Design review of the part built by this model. Coordinates are the model's own, in mm. Coordinates: 2 decimals unless noted, no trailing zeros. Order: outer loops, then holes, each group sorted by start corner. A loop starts at its lowest first (then second) coordinate and runs counter-clockwise, first axis right, second up.
from build123d import *

# Parameters (mm, degrees)
SKETCH_1_W          = 6.5
SKETCH_1_H          = 2
CUT_EXTRUDE_1_DEPTH = 1.5
CHAMFER_1_SIZE      = 0.75
CHAMFER_2_SIZE      = 0.6
CHAMFER_2_SIZE2     = 0.346410161
FILLET_1_R          = 0.1


with BuildPart() as part:
    # Эскиз1 → Повернуть1 (revolve)
    with BuildSketch(Plane(origin=(0, 0, 0), x_dir=(-1, 0, 0), z_dir=(0, 0, -1))):
        with Locations((-3.25, 1)):
            Rectangle(SKETCH_1_W, SKETCH_1_H)
    revolve(axis=Axis((6.5, 0, 0), (-1, 0, 0)))

    # Эскиз2 → Вырез-Вытянуть1 (cut)
    with BuildSketch(Plane.ZY):
        Polygon((1.154700538, 0), (0.577350269, 1), (-0.577350269, 1), (-1.154700538, 0), (-0.577350269, -1), (0.577350269, -1), align=None)
    extrude(amount=-CUT_EXTRUDE_1_DEPTH, mode=Mode.SUBTRACT)

    # Фаска1
    chamfer_1_edges = [part.edges().sort_by_distance(p)[0] for p in [
        (6.5, -2, 0),
    ]]
    chamfer(chamfer_1_edges, length=CHAMFER_1_SIZE)

    # Фаска2
    chamfer_2_edges = [part.edges().sort_by_distance(p)[0] for p in [
        (0, -2, 0),
    ]]
    chamfer_2_side = [part.faces().sort_by_distance(p)[0] for p in [
        (0, -1.943431458, 0),
    ]]
    chamfer(chamfer_2_edges, length=CHAMFER_2_SIZE, length2=CHAMFER_2_SIZE2, reference=chamfer_2_side[0])

    # Скругление1
    fillet_1_edges = [part.edges().sort_by_distance(p)[0] for p in [
        (1.5, -0.5, 0.866025404),
        (1.5, -1, 0),
        (1.5, -0.5, -0.866025404),
        (1.5, 0.5, -0.866025404),
        (1.5, 1, 0),
        (1.5, 0.5, 0.866025404),
        (0, -0.5, 0.866025404),
        (0, 0.5, 0.866025404),
        (0, 1, 0),
        (0, 0.5, -0.866025404),
        (0, -0.5, -0.866025404),
        (0, -1, 0),
        (0, -1.4, 0),
    ]]
    fillet(fillet_1_edges, radius=FILLET_1_R)


solid = part.part
1. Mouldability with a two-part tool opening along Y and no side actions: class faces 1 (the cylindrical face through (3, 0, 2)), 2 (the flat face through (0.74, -0.49, -0.87)), 3 (the flat face through (6.5, 0, 0)), 4 (the flat face through (0.74, 0.51, -0.86)) as pulls with the +Y half, pulls with the -Y half, needs draft (parallel to the pull), parting line crosses it, or undercut.
2. Add section C-C (x = 3). Give the boundary of the cut face in (y, z).
3. To check wall thickness, follow line 1 (Y direction, x = 1.25, z = -0.1); line 2 (Z direction, x = 0.5, y = -0.6); line 3 (X direction, y = 0.7, z = -0.65). State the ranges of each line that lie inside material, in increasing order.
4. Add section A-A (x = 0.75). Give the boundary of the cut face in (y, z).
5. Add section B-B (z = 0). Give the boundary of the cut face in (x, y), and give its area (3 significant figures).
6. Insertion check: pin 1 (1.5 mm diameter, centred on x = 5.5, y = 1, fed in from -Z); pin 2 (2 mm diameter, centred on x = 5, y = -1.5, fed in from +Z). Each pin has a flat end and moves straight along its axis. Give the tip position at first contact, or say it passes through.
Solution:
1. face 1: parting line crosses it
1. face 2: undercut
1. face 3: needs draft
1. face 4: undercut
2. outline: circle Ø4 at (0, 0)
3. line 1: y = -2 to -1, 1 to 2
3. line 2: z = -1.91 to -0.81, 0.81 to 1.91
3. line 3: x = 1.5 to 6.5
4. outline: circle Ø4 at (0, 0); hole (-1, -0.58) - (0, -1.15) - (1, -0.58) - (1, 0.58) - (0, 1.15) - (-1, 0.58) - close
5. outline: (0, -1.37) arc R0.1 ccw to (0.01, -1.42) - (0.35, -2) - (5.75, -2) - (6.5, -1.25) - (6.5, 1.25) - (5.75, 2) - (0.35, 2) - (0.01, 1.42) arc R0.1 ccw to (0, 1.37) - (0, 1.1) arc R0.1 ccw to (0.1, 1) - (1.4, 1) arc R0.1 cw to (1.5, 0.9) - (1.5, -0.9) arc R0.1 cw to (1.4, -1) - (0.1, -1) arc R0.1 ccw to (0, -1.1) - close
5. area: 22.2 mm2
6. pin 1: stops at z = -1.98
6. pin 2: stops at z = 1.94
